```python
from build123d import *

# Parameters (mm, degrees)
SKETCH1_W           = 65
SKETCH1_H           = 32
SKETCH1_R           = 2.5
BOSS_EXTRUDE1_DEPTH = 4
SKETCH2_W           = 65
SKETCH2_H           = 15
BOSS_EXTRUDE2_DEPTH = 2
CUT_EXTRUDE2_DEPTH  = 41.552435192


with BuildPart() as part:
    # Sketch1 → Boss-Extrude1 (new body)
    with BuildSketch(Plane(origin=(0, 0, 0), x_dir=(1, 0, 0), z_dir=(0, 1, 0))):
        Rectangle(SKETCH1_W, SKETCH1_H)
        with Locations(Location((-16, 10, 0), (0, 0, 270))):
            Circle(SKETCH1_R, mode=Mode.SUBTRACT)
        with Locations(Location((16, 10, 0), (0, 0, 270))):
            Circle(SKETCH1_R, mode=Mode.SUBTRACT)
        with Locations(Location((-16, -10, 0), (0, 0, 270))):
            Circle(SKETCH1_R, mode=Mode.SUBTRACT)
        with Locations(Location((16, -10, 0), (0, 0, 270))):
            Circle(SKETCH1_R, mode=Mode.SUBTRACT)
    extrude(amount=BOSS_EXTRUDE1_DEPTH)

    # Sketch2 → Boss-Extrude2 (add)
    with BuildSketch(Plane(origin=(0, 4, 0), x_dir=(1, 0, 0), z_dir=(0, 1, 0))):
        Rectangle(SKETCH2_W, SKETCH2_H)
    extrude(amount=BOSS_EXTRUDE2_DEPTH)

    # Sketch3 → Cut-Extrude2 (cut, through all)
    with BuildSketch(Plane.XY.offset(7.5)):
        Polygon((-32.5, 6), (-32.5, 4), (-32.1, 5.4), (-31.3, 6), align=None)
        Polygon((-30.3, 6), (-29.5, 5.4), (-29.1, 4), (-27.5, 4), (-27.1, 5.4), (-26.3, 6), align=None)
        Polygon((32.5, 6), (29.7, 6), (30.5, 5.4), (30.9, 4), (32.5, 4), align=None)
        Polygon((-24.1, 6), (-25.3, 6), (-24.5, 5.4), (-24.1, 4), (-22.5, 4), (-22.1, 5.4), (-21.3, 6), align=None)
        Polygon((-20.3, 6), (-19.5, 5.4), (-19.1, 4), (-17.5, 4), (-17.1, 5.4), (-16.3, 6), align=None)
        Polygon((-15.3, 6), (-14.5, 5.4), (-14.1, 4), (-12.5, 4), (-12.1, 5.4), (-11.3, 6), align=None)
        Polygon((-10.3, 6), (-9.5, 5.4), (-9.1, 4), (-7.5, 4), (-7.1, 5.4), (-6.3, 6), align=None)
        Polygon((-5.3, 6), (-4.5, 5.4), (-4.1, 4), (-2.5, 4), (-2.1, 5.4), (-1.3, 6), align=None)
        Polygon((-0.3, 6), (0.5, 5.4), (0.9, 4), (2.5, 4), (2.9, 5.4), (3.7, 6), align=None)
        Polygon((4.7, 6), (5.5, 5.4), (5.9, 4), (7.5, 4), (7.9, 5.4), (8.7, 6), align=None)
        Polygon((9.7, 6), (10.5, 5.4), (10.9, 4), (12.5, 4), (12.9, 5.4), (13.7, 6), align=None)
        Polygon((14.7, 6), (15.5, 5.4), (15.9, 4), (17.5, 4), (17.9, 5.4), (18.7, 6), align=None)
        Polygon((19.7, 6), (20.5, 5.4), (20.9, 4), (22.5, 4), (22.9, 5.4), (23.7, 6), align=None)
        Polygon((24.7, 6), (25.5, 5.4), (25.9, 4), (27.5, 4), (27.9, 5.4), (28.7, 6), align=None)
    extrude(amount=-CUT_EXTRUDE2_DEPTH, mode=Mode.SUBTRACT)


solid = part.part
```
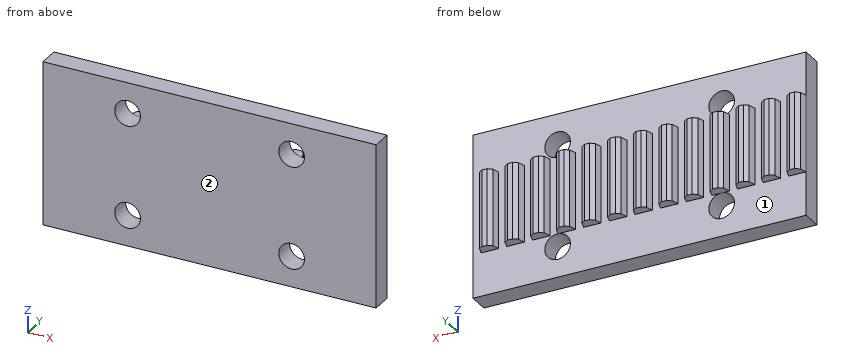
Can you work these out from the model? Positions are in its coordinate system, mm. Face numbers are marked on the shaded views. A direction names the side the tool comes from. Give positions to 0.01 mm unless a question says otherwise; leave off trailing zeros. Loops run counter-clockwise (first coordinate to the right, second up) from the corner with the lowest first, then second, coordinate; pieces in that order, holes last. Notation, with made-up numbers: M 72,30.25 L 93,30.25 A18 cw 93,52.25 Z; hole C 42.5,-29 d4. An arc over 180 degrees is marked long. Answer in a Markdown table with one row per item.
1. Which directions (+Z, -Z, +X, -X, +Y, -Y) give clear straight access to the entire face, cutting with the end or side of a thin tool? Please do the marked faces 1 and 2.
Taken from the geometry:
| item | result |
|---|---|
| face 1 | +Y |
| face 2 | +Z, -Z, +X, -X, -Y |
2. For pin 1 Ø1.6 at (x, y) = (-11, 5) entering from +Z; pin 2 Ø1 at (x, y) = (-16.5, 5.5) entering from -Z; pin 3 Ø3 at (x, z) = (11.5, -12) entering from -Y; pin 4 Ø8 at (x, z) = (-3, 12) entering from +Y, each with a flat end and sliding along its axis, tell me the tip position at first contact or that it passes through.
Taken from the geometry:
| item | result |
|---|---|
| pin 1 | stops at z = 7.5 |
| pin 2 | stops at z = -7.5 |
| pin 3 | stops at y = 0 |
| pin 4 | stops at y = 4 |
3. Suppose I cut it at A-A on z = -10. Write out the boundary of the cut face in (x, y).
Taken from the geometry:
| item | result |
|---|---|
| outline | M -32.5,0 L -18.5,0 L -18.5,4 L -32.5,4 Z; M -13.5,0 L 13.5,0 L 13.5,4 L -13.5,4 Z; M 18.5,0 L 32.5,0 L 32.5,4 L 18.5,4 Z |
4. Suppose I cut it at C-C on x = 11.5. Write out the boundary of the cut face in (y, z), plus the area to 3 significant figures.
Taken from the geometry:
| item | result |
|---|---|
| outline | M 0,-16 L 4,-16 L 4,16 L 0,16 Z |
| area | 128 mm² |
5. Suppose I cut it at B-B on y = 2. Write out the boundary of the cut face in (x, z), plus the area to 3 significant figures.
Taken from the geometry:
| item | result |
|---|---|
| outline | M -32.5,-16 L 32.5,-16 L 32.5,16 L -32.5,16 Z; hole C -16,-10 d5; hole C -16,10 d5; hole C 16,-10 d5; hole C 16,10 d5 |
| area | 2,000 mm² |
6. If I drill on line 1 along X through (y, z) = (2.15, -10); line 2 along Z through (x, y) = (-16, 1.95); line 3 along Y through (x, z) = (21.5, -6), over which ranges is the centre line in solid material (lowest first)?
Taken from the geometry:
| item | result |
|---|---|
| line 1 | x = -32.5 to -18.5, -13.5 to 13.5, 18.5 to 32.5 |
| line 2 | z = -16 to -12.5, -7.5 to 7.5, 12.5 to 16 |
| line 3 | y = 0 to 4 |
